Autodesk Inventor part; units mm, degrees
ref_plane "YZ Plane" through (0, 0, 0) normal (1, 0, 0) x (0, 1, 0)
ref_plane "XZ Plane" through (0, 0, 0) normal (0, 1, 0) x (-1, 0, 0)
ref_plane "XY Plane" through (0, 0, 0) normal (0, 0, 1) x (1, 0, 0)
sketch "Skizze1" plane through (0, 0, 0) normal (1, 0, 0) x (0, 1, 0)
  line L0 (-6, 5) -> (-10.5, 0.5)
  line L1 (-10.5, 0) -> (-3, 0)
  line L2 (0, 3) -> (0, 8)
  line L3 (-10.5, 0.5) -> (-10.5, 0)
  line L4 (0, 8) -> (5, 13)
  line L5 (0, 8) -> (0, 19.5) construction
  circle A0 centre (0, 19.5) radius 0.5
  line L6 (-5, 13) -> (-5, 24.5)
  line L7 (-5, 24.5) -> (5, 24.5)
  line L8 (5, 24.5) -> (5, 13)
  line L9 (0, 3) -> (-3, 0)
  line L10 (-5, 13) -> (-6, 12)
  line L11 (-6, 12) -> (-6, 5)
  line L12 (5, 13) -> (-5, 13) construction
  point P0 (0, 0)
  dimension "d40" = 0.5
  dimension "d41" = 10.5
  dimension "d44" = 1
  dimension "d56" = 5
  dimension "d58" = 19.5
  dimension "d59" = 10
  dimension "d60" = 45
  dimension "d61" = 8
  dimension "d62" = 3
  dimension "d63" = 45
  dimension "d67" = 1
extrude "Extrusion1" add sketch "Skizze1" along normal mid plane 67
sketch "Skizze6" plane through (0, 0, 0) normal (0, 1, 0) x (-1, 0, 0)
  line L0 (33.5, 0.5) -> (-33.5, 0.5)
  line L1 (-33.5, 5) -> (-33.5, 0.5)
  line L2 (33.5, 0.5) -> (33.5, 5)
  line L3 (-29.5, 6) -> (29.5, 6)
  line L4 (29.5, 6) -> (29.5, 36)
  line L5 (29.5, 36) -> (-29.5, 36)
  line L6 (-29.5, 36) -> (-29.5, 6)
  line L7 (0, -7.1) -> (0, 42.6)
  line L8 (33.5, 0) -> (-33.5, 0)
  line L9 (-33.5, 0) -> (33.5, 0)
  point P0 (0, 0)
  point P1 (-33, 10)
  point P2 (33, 10)
  dimension "d45" = 4
  dimension "d46" = 30
  dimension "d50" = 6
extrude "Extrusion4" cut sketch "Skizze6" along normal through all both and the other way through all
sketch "Skizze3" plane through (-33.5, 0, 0) normal (-1, 0, 0) x (0, 0, 1)
  line L0 (8, 0) -> (3, 0)
  line L1 (0, -3) -> (0, -10.5)
  line L2 (0.5, -10.5) -> (5, -6)
  line L3 (0, -10.5) -> (0, 0) construction
  line L4 (0, 8.1) -> (0, -13.6)
  line L5 (0, -10.5) -> (0.5, -10.5)
  line L6 (13, 5) -> (8, 0)
  line L7 (13, -5) -> (24.5, -5)
  line L8 (24.5, -5) -> (24.5, 5)
  line L9 (24.5, 5) -> (13, 5)
  circle A0 centre (19.5, 0) radius 0.5
  line L10 (3, 0) -> (0, -3)
  line L11 (5, -6) -> (12, -6)
  line L12 (12, -6) -> (13, -5)
hole "Bohrung1" at (-33.5, 0, 19.5) direction (1, 0, 0) diameter 4.05 end through all
sketch "Skizze4" plane through (-33.5, 0, 0) normal (-1, 0, 0) x (0, 0, 1)
  line L0 (8, 0) -> (0, 0)
  line L1 (0, 8.1) -> (0, -13.6)
  point P0 (29, 0)
  point P1 (11, -1)
  dimension "d38" = 11
  dimension "d69" = 1
hole "Bohrung2" at (-33.5, -1, 11) direction (1, 0, 0) diameter 2.459 end through all
fillet "Rundung1" [suppressed]
fillet "Rundung2" radius 5 4 edges at (31.5, -5, 24.5) (31.5, 5, 24.5) (-31.5, 5, 24.5) (-31.5, -5, 24.5)
fillet "Rundung5" radius 4 2 edges at (31.5, 5, 13) (-31.5, 5, 13)
fillet "Rundung7" radius 3 6 edges at (-31.5, 0, 8) (31.5, 0, 8) (31.5, -6, 12) (31.5, -5, 13) (-31.5, -6, 12) (-31.5, -5, 13)
fillet "Rundung8" radius 0.36 2 edges at (0, -10.5, 0.5) (0, -10.5, 0)
properties part number "Chip Schaufel" material "Aluminium 6061"
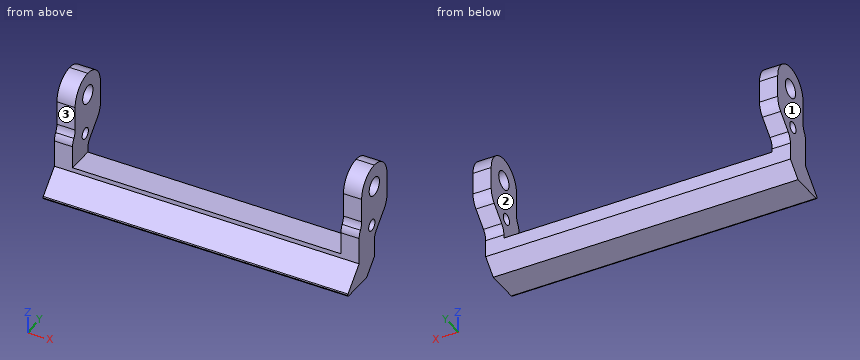
Here's how the part is built. I have some questions about the finished solid (model axes, mm). Face numbers are marked on the shaded views. A direction names the side the tool comes from. Coordinates: 2 decimals unless noted, no trailing zeros. Loops run counter-clockwise (first coordinate to the right, second up) from the corner with the lowest first, then second, coordinate; pieces in that order, holes last. Notation, with made-up numbers: (-7, 52.25) - (3, 52.25) arc R10 ccw to (3, 62.25) - close; hole circle Ø3 at (-0.75, 5.25). An arc over 180 degrees is marked (long way). Answer as CSV lines item,"result".
Q1. If I drill on L1, parallel to X at y = 1, z = 10; L2, parallel to Z at x = -31, y = -1; L3, parallel to Y at x = -32.7, z = 19.5 (3 decimals), over which ranges is the centre line in solid material (lowest first)? Write a range as [from, to].
Response:
L1,"[-33.5, -29.5], [29.5, 33.5]"
L2,"[2, 9.77], [12.23, 17.74], [21.26, 24.4]"
L3,"[-5, -2.025], [2.025, 5]"
Q2. If we section it at D-D, the plane y = -4: Write out the boundary of the cut face in (x, z), and give its area (3 significant figures).
Response:
outline,"(-33.5, 0) - (33.5, 0) - (33.5, 22.5) - (29.5, 22.5) - (29.5, 6) - (-29.5, 6) - (-29.5, 22.5) - (-33.5, 22.5) - close"
area,"534 mm2"
Q3. For pin 1 (3 mm diameter, centred on x = -6, z = 7, fed in from -Y); pin 2 (2 mm diameter, centred on x = -31, z = 18, fed in from -Y); pin 3 (2 mm diameter, centred on x = 8.5, y = 0.5, fed in from +Z); pin 4 (2 mm diameter, centred on y = -1, z = 11, fed in from +X), each with a flat end and sliding along its axis, tell me the tip position at first contact or that it passes through.
Response:
pin 1,"y = -6"
pin 2,"y = -5"
pin 3,"z = 6"
pin 4,"through"
Q4. For the marked faces 1, 2 and 3, which set-ups out of +Z, -Z, +X, -X, +Y, -Y let a thin tool reach every point of the face, with its end or its side?
Response:
face 1,"+Z, -Z, -X, +Y, -Y"
face 2,"+Z, +Y, -Y"
face 3,"+Z, +X, -X, -Y"
Q5. If we section it at C-C, the plane z = 23.25: Write out the boundary of the cut face in (x, y).
Response:
outline,"(-33.5, -3.31) - (-29.5, -3.31) - (-29.5, 3.31) - (-33.5, 3.31) - close; (29.5, -3.31) - (33.5, -3.31) - (33.5, 3.31) - (29.5, 3.31) - close"
Q6. If we section it at B-B, the plane x = 21.5: Write out the boundary of the cut face in (y, z), and give its area (3 significant figures).
Response:
outline,"(-10.5, 0.36) arc R0.36 ccw to (-10.14, 0) - (-3, 0) - (0, 3) - (0, 6) - (-6, 6) - (-6, 5) - (-10.39, 0.61) arc R0.36 ccw to start"
area,"43.8 mm2"
Q7. If we section it at A-A, the plane y = -1: Write out the boundary of the cut face in (x, z).
Response:
outline,"(-33.5, 2) - (33.5, 2) - (33.5, 9.77) - (29.5, 9.77) - (29.5, 6) - (-29.5, 6) - (-29.5, 9.77) - (-33.5, 9.77) - close; (-33.5, 12.23) - (-29.5, 12.23) - (-29.5, 17.74) - (-33.5, 17.74) - close; (-33.5, 21.26) - (-29.5, 21.26) - (-29.5, 24.4) - (-33.5, 24.4) - close; (29.5, 12.23) - (33.5, 12.23) - (33.5, 17.74) - (29.5, 17.74) - close; (29.5, 21.26) - (33.5, 21.26) - (33.5, 24.4) - (29.5, 24.4) - close"
